Build history of the part. All positions in model axes, mm. Give positions to 0.01 mm unless a question says otherwise; leave off trailing zeros. Write each loop counter-clockwise with the first axis right and the second up, starting at its lowest first coordinate (ties: lowest second). Pieces come first, ordered by that corner, then holes. Notation, with made-up numbers: (26.5, 43) -> (64.5, 43) arc R33 cw to (64.5, 78) -> close; hole circle Ø3 at (1, -24.75). An arc over 180 degrees is marked (long way). Put each result on its own line as item: value. Start each with the question number.
Item 1: Slice it at B-B, the plane z = 113. List the corners of the cut face in (x, y), plus the area to 3 significant figures.
Item 2: Flat gauge pin, fed straight in: pin 1 Ø6.5 at (x, z) = (75, 175.29) entering from -Y. Where does the tip first touch, or does it go through?
Item 3: Slice it at A-A, the plane x = 55. List the corners of the cut face in (y, z).
Item 4: Slice it at C-C, the plane y = 2.3. List the corners of the cut face in (x, z).
Item 5: Drill centre lines: line 1 along Z through (x, y) = (61.5, 1.6); line 2 along X through (y, z) = (2.75, -126); line 3 along Z through (x, y) = (77, 1.25). Where is each one in solid material? Low to high.
```python
from build123d import *

# Parameters (mm, degrees)
SKETCH1_R           = 2.55
SKETCH1_W           = 152
SKETCH1_H           = 99
SKETCH1_H_2         = 65
BOSS_EXTRUDE1_DEPTH = 3


with BuildPart() as part:
    # Sketch1 → Boss-Extrude1 (new body)
    with BuildSketch(Plane(origin=(0, 0, 0), x_dir=(1, 0, 0), z_dir=(0, 1, 0))):
        with BuildLine():
            Line((-80, -180), (80, -180))
            ThreePointArc((80, -180), (87.071067812, -177.071067812), (90, -170))
            Line((90, -170), (90, 170))
            ThreePointArc((90, 170), (87.071067812, 177.071067812), (80, 180))
            Line((80, 180), (-80, 180))
            ThreePointArc((-80, 180), (-87.071067812, 177.071067812), (-90, 170))
            Line((-90, 170), (-90, -170))
            ThreePointArc((-90, -170), (-87.071067812, -177.071067812), (-80, -180))
        make_face()
        with Locations(Location((-75, 175.287107213, 0), (0, 0, 270))):
            Circle(SKETCH1_R, mode=Mode.SUBTRACT)
        with Locations(Location((75, 175.287107213, 0), (0, 0, 270))):
            Circle(SKETCH1_R, mode=Mode.SUBTRACT)
        with Locations(Location((-75, -175.287107213, 0), (0, 0, 90))):
            Circle(SKETCH1_R, mode=Mode.SUBTRACT)
        with Locations(Location((75, -175.287107213, 0), (0, 0, 90))):
            Circle(SKETCH1_R, mode=Mode.SUBTRACT)
        with Locations((0, 120.5)):
            Rectangle(SKETCH1_W, SKETCH1_H, mode=Mode.SUBTRACT)
        with Locations((0, -137.5)):
            Rectangle(SKETCH1_W, SKETCH1_H_2, mode=Mode.SUBTRACT)
        with Locations((0, 11.5)):
            Rectangle(SKETCH1_W, SKETCH1_H, mode=Mode.SUBTRACT)
    extrude(amount=BOSS_EXTRUDE1_DEPTH)


solid = part.part
```
Values follow:
1. outline: (-90, 0) -> (-76, 0) -> (-76, 3) -> (-90, 3) -> close; (76, 0) -> (90, 0) -> (90, 3) -> (76, 3) -> close
1. area: 84.0 mm2
2. pin 1: y = 0
3. outline: (0, -180) -> (3, -180) -> (3, -170) -> (0, -170) -> close; (0, -71) -> (3, -71) -> (3, -61) -> (0, -61) -> close; (0, 38) -> (3, 38) -> (3, 105) -> (0, 105) -> close; (0, 170) -> (3, 170) -> (3, 180) -> (0, 180) -> close
4. outline: (-90, -170) arc R10 ccw to (-80, -180) -> (80, -180) arc R10 ccw to (90, -170) -> (90, 170) arc R10 ccw to (80, 180) -> (-80, 180) arc R10 ccw to (-90, 170) -> close; hole circle Ø5.1 at (-75, -175.29); hole circle Ø5.1 at (-75, 175.29); hole (-76, -170) -> (76, -170) -> (76, -71) -> (-76, -71) -> close; hole (-76, -61) -> (76, -61) -> (76, 38) -> (-76, 38) -> close; hole (-76, 105) -> (76, 105) -> (76, 170) -> (-76, 170) -> close; hole circle Ø5.1 at (75, -175.29); hole circle Ø5.1 at (75, 175.29)
5. line 1: -180 to -170, -71 to -61, 38 to 105, 170 to 180
5. line 2: -90 to -76, 76 to 90
5. line 3: -180 to -176.87, -173.71 to 173.71, 176.87 to 180
